Can you work these out from the drawing? Everything is in mm from the part's minimum corner. Coordinates: 2 decimals unless noted, no trailing zeros. Loops run counter-clockwise (first coordinate to the right, second up) from the corner with the lowest first, then second, coordinate; pieces in that order, holes last.
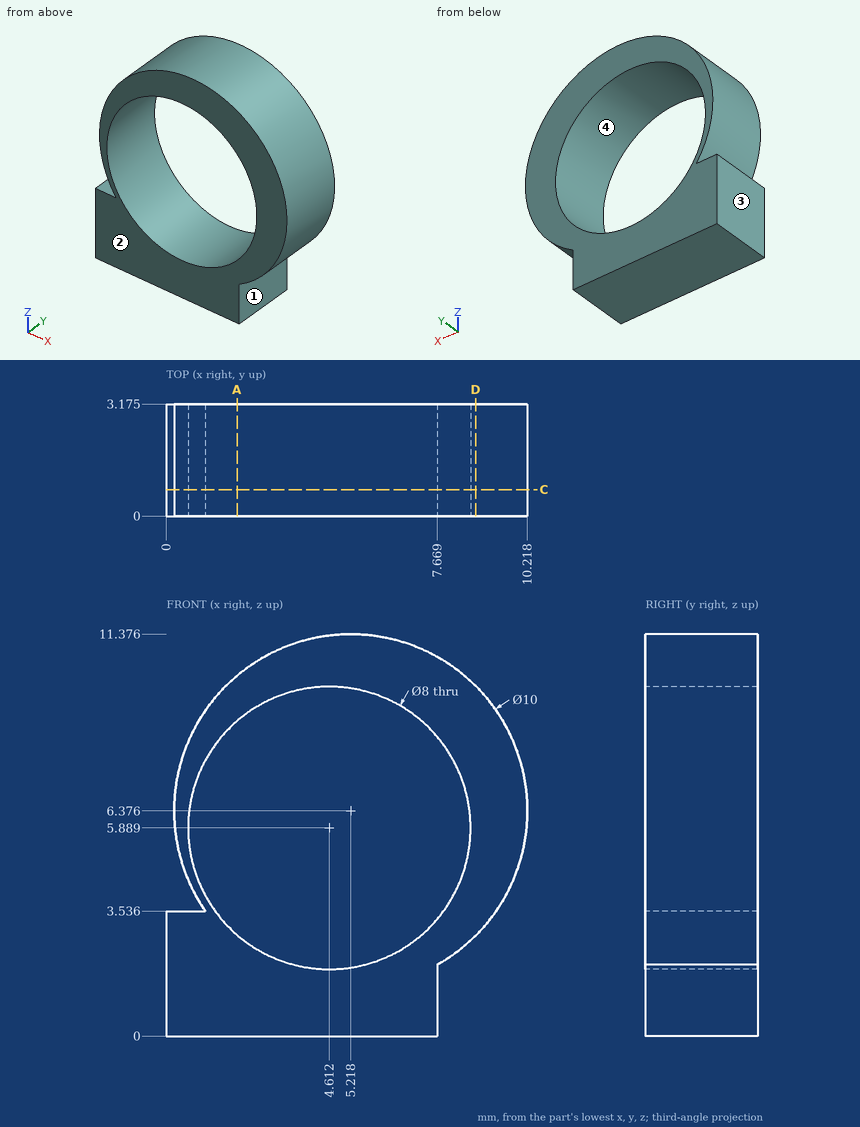
1) We'd pull the mould along X, two halves only. Please class the marked faces 1, 2, 3 and 4: released by +X, released by -X, zero draft, split by the parting line, or undercut.
2) Imagine slicing it at A-A on x = 2. List the corners of the cut face in (y, z) for me (1 decimal).
3) Imagine slicing it at C-C on y = 0.75. List the corners of the cut face in (x, z) for me (1 decimal).
4) If I drill on L1, parallel to Z at x = 4.5, y = 1.1; L2, parallel to X at y = 3, z = 8 (1 decimal); L3, parallel to Z at x = 3, y = 0.2, over which ranges is the centre line in solid material (lowest first)?
5) Imagine slicing it at D-D on x = 8.75. List the corners of the cut face in (y, z) for me (1 decimal), plus the area to 3 significant figures.
6) Will these pins go through, and if not, where does the flat tip stop? pin 1 (1.5 mm diameter, centred on y = 0.5, z = 3, fed in from +X); pin 2 (5 mm diameter, centred on x = 4.61, z = 5.89, fed in from -Y); pin 3 (1.6 mm diameter, centred on y = 1, z = 1, fed in from +X); pin 4 (1.5 mm diameter, centred on y = 2.5, z = 9, fed in from +X).
Solved:
1. face 1: released by +X
1. face 2: zero draft
1. face 3: released by -X
1. face 4: undercut
2. outline: (0, 0) - (3.2, 0) - (3.2, 2.9) - (0, 2.9) - close; (0, 8.9) - (3.2, 8.9) - (3.2, 10.2) - (0, 10.2) - close
3. outline: (0, 0) - (7.7, 0) - (7.7, 2) arc R5 ccw (long way) to (1.1, 3.5) - (0, 3.5) - close; hole circle Ø8 at (4.6, 5.9)
4. L1: z = 0 to 1.89, 9.89 to 11.32
4. L2: x = 0.5 to 1.2, 8 to 9.9
4. L3: z = 0 to 2.23, 9.55 to 10.86
5. outline: (0, 2.8) - (3.2, 2.8) - (3.2, 9.9) - (0, 9.9) - close
5. area: 22.5 mm2
6. pin 1: stops at x = 9.47
6. pin 2: passes through
6. pin 3: stops at x = 7.67
6. pin 4: stops at x = 9.85
